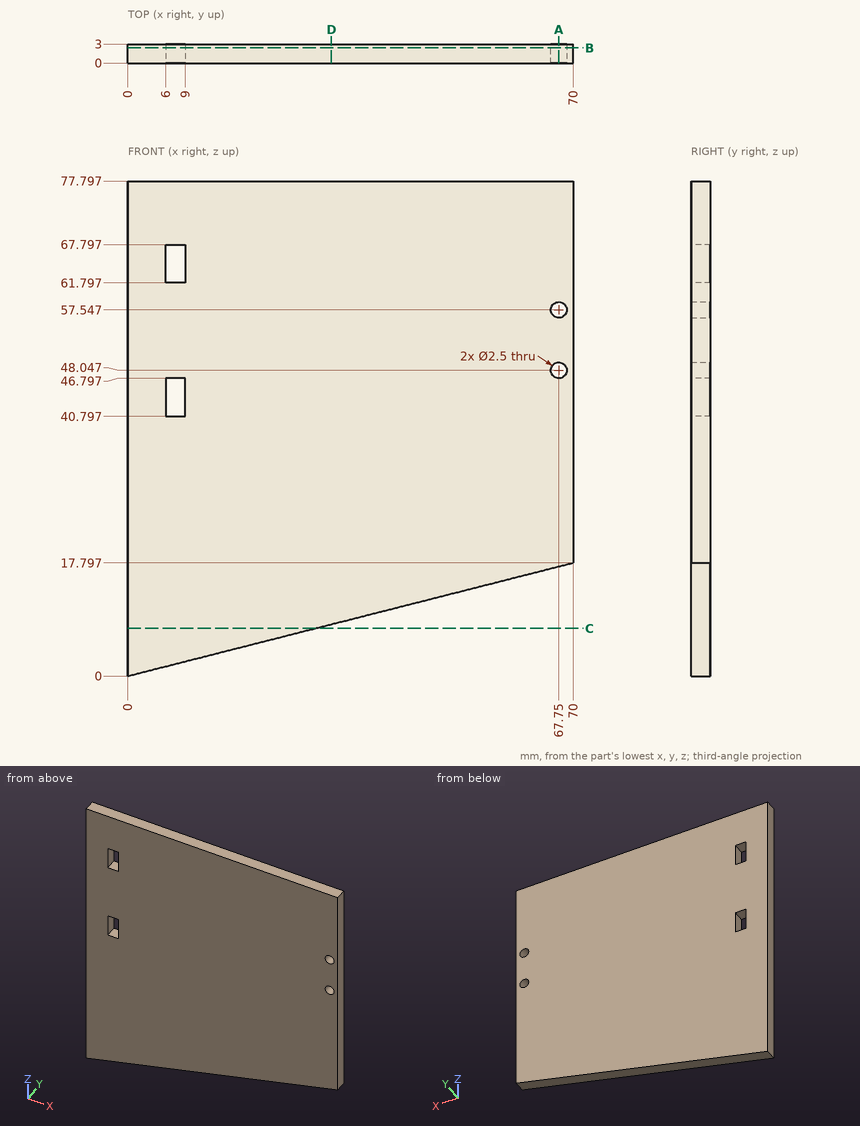
Could you check a few things on this drawing? It's one solid part, dimensions in mm from its lowest x, y, z. Give positions to 0.01 mm unless a question says otherwise; leave off trailing zeros. Order: outer loops, then holes, each group sorted by start corner. A loop starts at its lowest first (then second) coordinate and runs counter-clockwise, first axis right, second up. Notation, with made-up numbers: (83.5, 85) - (126.5, 85) arc R23 ccw to (126.5, 99) - close; hole circle Ø1 at (-40, -5). An arc over 180 degrees is marked (long way). One line per question, with ' | ' between items. Start each with the question number.
Item 1: I want a section at D-D on x = 32. Write out the boundary of the cut face in (y, z) (1 decimal).
Item 2: I want a section at C-C on z = 7.5. Write out the boundary of the cut face in (x, y).
Item 3: I'm going to push a flat-ended pin straight in: pin 1 Ø2 at (x, z) = (67.75, 48.05) entering from +Y. Where does the tip first touch, or does it pass through?
Item 4: I want a section at B-B on y = 2.4. Write out the boundary of the cut face in (x, z), then the cut area to 3 significant figures.
Item 5: I need wall thicknesses on probe 1 along X at (y, z) = (0.65, 46); probe 2 along Z at (x, y) = (67.75, 1.8) (1 decimal); probe 3 along Z at (x, y) = (54, 1.7). Which ranges of each line are inside material? Lowest first, please. Write a range as [from, to].
Item 6: I want a section at A-A on x = 67.75. Write out the boundary of the cut face in (y, z) (1 decimal), then the cut area to 3 significant figures.
Verdict:
1) outline: (0, 8.1) - (3, 8.1) - (3, 77.8) - (0, 77.8) - close
2) outline: (0, 0) - (29.5, 0) - (29.5, 3) - (0, 3) - close
3) pin 1: through
4) outline: (0, 0) - (70, 17.8) - (70, 77.8) - (0, 77.8) - close; hole (6, 40.8) - (9, 40.8) - (9, 46.8) - (6, 46.8) - close; hole (6, 61.8) - (9, 61.8) - (9, 67.8) - (6, 67.8) - close; hole circle Ø2.5 at (67.75, 48.05); hole circle Ø2.5 at (67.75, 57.55) | area: 4,780 mm^2
5) probe 1: [0, 6], [9, 70] | probe 2: [17.2, 46.8], [49.3, 56.3], [58.8, 77.8] | probe 3: [13.73, 77.8]
6) outline: (0, 17.2) - (3, 17.2) - (3, 46.8) - (0, 46.8) - close; (0, 49.3) - (3, 49.3) - (3, 56.3) - (0, 56.3) - close; (0, 58.8) - (3, 58.8) - (3, 77.8) - (0, 77.8) - close | area: 167 mm^2
